Read the model definition and answer for the solid it produces. Units are mm, in the model's axes. A direction names the side the tool comes from. Round coordinates to 2 decimals unless told otherwise and drop trailing zeros. Order: outer loops, then holes, each group sorted by start corner. A loop starts at its lowest first (then second) coordinate and runs counter-clockwise, first axis right, second up. Notation, with made-up numbers: (17.25, 77) - (57.25, 77) arc R22 ccw to (57.25, 94) - close; hole circle Ø11 at (17.5, 58.5). An arc over 180 degrees is marked (long way). Answer as a JSON object with one key per item and string values. Group by question number.
Q1. A cutting plane is placed at B-B on y = 7.5. Determine the outline of the cut face in (x, z), and give its area (3 significant figures).
Q2. Consider line 1 (X direction, y = 6.5, z = 1.75); line 2 (Y direction, x = 6, z = 1); line 3 (X direction, y = 0, z = 1.55). Determine where each line is inside the solid, lowest interval first.
Q3. A tool of negligible diameter and unlimited length cuts with its end or side. For faces 1 (the flat face through (11.033, 1.821, 0.986)), 2 (the flat face through (-10.2, 20, 1)), 3 (the flat face through (18, 18.5, 1)), from which of +Z, -Z, +X, -X, +Y, -Y can it reach the whole face along a straight path? Write none if from no direction.
Q4. A cutting plane is placed at D-D on y = 2.5. Determine the outline of the cut face in (x, z).
Q5. A cutting plane is placed at A-A on x = -9. Determine the outline of the cut face in (y, z), and give its area (3 significant figures).
Q6. A cutting plane is placed at C-C on z = 0.4. Count the separate pieces of the cut face and the enclosed holes in it, and give its area (3 significant figures).
Q7. Given pin 1 Ø0.6 at (y, z) = (20.5, 1) entering from +X; pin 2 Ø1 at (x, z) = (-18.5, 1) entering from -Y, each flat-ended and moving along its own axis, determine where each tip first touches the part or whether it passes through.
Q8. The mould has two halves that part along Y. Classify faces 4 (the cylindrical face through (-2.563, 6.677, 1.014)), 5 (the flat face through (9.8, -20, 1)), 6 (the cylindrical face through (10.87, 17.45, 0.99)), 7 (the cylindrical face through (3.465, 13.703, 1.014)): pulls with the +Y half, pulls with the -Y half, needs draft (parallel to the pull), parting line crosses it, or undercut.
```python
from build123d import *

# Parameters (mm, degrees)
SKETCH_1_W          = 50
SKETCH_1_H          = 37
EXTRUDE_1_DEPTH     = 2
SKETCH_2_W          = 20
SKETCH_2_H          = 2
EXTRUDE_2_DEPTH     = 4
SKETCH_3_R          = 1.05
CUT_EXTRUDE_1_DEPTH = 3
CUT_EXTRUDE_3_DEPTH = 10
FILLET_1_R          = 1.5


with BuildPart() as part:
    # 草图1 → 凸台-拉伸1 (new body)
    with BuildSketch(Plane.XY):
        Rectangle(SKETCH_1_W, SKETCH_1_H)
    extrude(amount=EXTRUDE_1_DEPTH)

    # 草图2 → 凸台-拉伸2 (add)
    with BuildSketch(Plane(origin=(0, 18.5, 0), x_dir=(1, 0, 0), z_dir=(0, 1, 0))):
        with Locations((-0.2, -1)):
            Rectangle(SKETCH_2_W, SKETCH_2_H)
    extrude_2 = extrude(amount=EXTRUDE_2_DEPTH)

    # 镜向1: 凸台-拉伸2 across plane
    add(extrude_2.mirror(Plane.ZX))

    # 草图3 → 切除-拉伸1 (cut)
    with BuildSketch(Plane(origin=(0, 0, 0), x_dir=(-1, 0, 0), z_dir=(0, 0, -1))):
        with Locations((11.25, 18.5)):
            Circle(SKETCH_3_R)
        with Locations((-10.85, 18.5)):
            Circle(SKETCH_3_R)
        with Locations((-10.85, -18.5)):
            Circle(SKETCH_3_R)
        with Locations((11.25, -18.5)):
            Circle(SKETCH_3_R)
    extrude(amount=-CUT_EXTRUDE_1_DEPTH, mode=Mode.SUBTRACT)

    # 草图4 → 切除-拉伸3 (cut)
    with BuildSketch(Plane(origin=(0, 0, 0), x_dir=(-1, 0, 0), z_dir=(0, 0, -1))):
        Polygon((-21, 14.5), (-21, -11.94249803), (-1.851984185, 14.5), align=None)
        Polygon((-19.148015815, -14.5), (-1.5, -14.5), (-1.5, 9.871069459), align=None)
        Polygon((1.5, 9.871069459), (1.5, -14.5), (19.148015815, -14.5), align=None)
        Polygon((1.851984185, 14.5), (21, -11.94249803), (21, 14.5), align=None)
    extrude(amount=-CUT_EXTRUDE_3_DEPTH, mode=Mode.SUBTRACT)

    # 圆角1
    fillet_1_edges = [part.edges().sort_by_distance(p)[0] for p in [
        (-1.851984185, 14.5, 1),
        (-21, 14.5, 1),
        (-21, -11.94249803, 1),
        (1.851984185, 14.5, 1),
        (21, -11.94249803, 1),
        (21, 14.5, 1),
        (25, -18.5, 1),
        (-25, -18.5, 1),
        (-25, 18.5, 1),
        (25, 18.5, 1),
        (1.5, 9.871069459, 1),
        (1.5, -14.5, 1),
        (19.148015815, -14.5, 1),
        (-1.5, 9.871069459, 1),
        (-19.148015815, -14.5, 1),
        (-1.5, -14.5, 1),
    ]]
    fillet(fillet_1_edges, radius=FILLET_1_R)


solid = part.part
```
Result set:
{
 "1": {"outline": "(-25, 0) - (-21, 0) - (-21, 2) - (-25, 2) - close; (-6.92, 0) - (6.92, 0) - (6.92, 2) - (-6.92, 2) - close; (21, 0) - (25, 0) - (25, 2) - (21, 2) - close", "area": "43.7 mm²"},
 "2": {"line 1": "x = -25 to -21, -7.65 to -3.82, -2.18 to 2.18, 3.82 to 7.65, 21 to 25", "line 2": "y = -22.5 to -14.5, 3.66 to 8.77, 14.5 to 22.5", "line 3": "x = -25 to -21, -12.35 to -8.65, -1.5 to 1.5, 8.65 to 12.35, 21 to 25"},
 "3": {"face 1": "+Z, -Z", "face 2": "+Z, -Z, -X, +Y", "face 3": "+Z, -Z, +X, +Y"},
 "4": {"outline": "(-25, 0) - (-21, 0) - (-21, 2) - (-25, 2) - close; (-10.54, 0) - (-6.84, 0) - (-6.84, 2) - (-10.54, 2) - close; (-1.5, 0) - (1.5, 0) - (1.5, 2) - (-1.5, 2) - close; (6.84, 0) - (10.54, 0) - (10.54, 2) - (6.84, 2) - close; (21, 0) - (25, 0) - (25, 2) - (21, 2) - close"},
 "5": {"outline": "(-22.5, 0) - (-14.5, 0) - (-14.5, 2) - (-22.5, 2) - close; (-0.49, 0) - (4.63, 0) - (4.63, 2) - (-0.49, 2) - close; (14.5, 0) - (22.5, 0) - (22.5, 2) - (14.5, 2) - close", "area": "42.2 mm²"},
 "6": {"separate pieces": "1", "enclosed holes": "4", "area": "1,090 mm²"},
 "7": {"pin 1": "stops at x = 9.8", "pin 2": "stops at y = -18.5"},
 "8": {"face 4": "undercut", "face 5": "needs draft", "face 6": "pulls with the +Y half", "face 7": "undercut"}
}
